Input: part model. Units: mm. Frame: model coordinates. Coordinates: 2 decimals unless noted, no trailing zeros. Order: outer loops, then holes, each group sorted by start corner. A loop starts at its lowest first (then second) coordinate and runs counter-clockwise, first axis right, second up. Notation, with made-up numbers: (-6.5, 14) -> (42.5, 14) arc R23 cw to (42.5, 30) -> close; hole circle Ø11 at (-6.5, -29). An arc over 180 degrees is marked (long way). Write each question's results on one line, items separated by ' | '.
```python
from build123d import *

# Parameters (mm, degrees)
F0_R     = 2.5527
F1_DEPTH = 6


with BuildPart() as f1:
    # F0 (on Right) → F1 (new body)
    with BuildSketch(Plane.YZ):
        with BuildLine():
            Line((-63.5, 177.8), (-114.3, 177.8))
            Line((-114.3, 177.8), (-114.3, 0))
            Line((-114.3, 0), (114.3, 0))
            Line((114.3, 0), (114.3, 177.8))
            Line((114.3, 177.8), (63.5, 177.8))
            ThreePointArc((63.5, 177.8), (0, 151.497439), (-63.5, 177.8))
        make_face()
        with Locations((-101.6, 12.7)):
            Circle(F0_R, mode=Mode.SUBTRACT)
        with Locations((-88.9, 12.7)):
            Circle(F0_R, mode=Mode.SUBTRACT)
        with Locations((-76.2, 12.7)):
            Circle(F0_R, mode=Mode.SUBTRACT)
        with Locations((-63.5, 12.7)):
            Circle(F0_R, mode=Mode.SUBTRACT)
        with Locations((-101.6, 25.4)):
            Circle(F0_R, mode=Mode.SUBTRACT)
        with Locations((-101.6, 38.1)):
            Circle(F0_R, mode=Mode.SUBTRACT)
        with Locations((-50.8, 12.7)):
            Circle(F0_R, mode=Mode.SUBTRACT)
        with Locations((-38.1, 12.7)):
            Circle(F0_R, mode=Mode.SUBTRACT)
        with Locations((-25.4, 12.7)):
            Circle(F0_R, mode=Mode.SUBTRACT)
        with Locations((-12.7, 12.7)):
            Circle(F0_R, mode=Mode.SUBTRACT)
        with Locations((-101.6, 50.8)):
            Circle(F0_R, mode=Mode.SUBTRACT)
        with Locations((-101.6, 63.5)):
            Circle(F0_R, mode=Mode.SUBTRACT)
        with Locations((-101.6, 76.2)):
            Circle(F0_R, mode=Mode.SUBTRACT)
        with Locations((0, 12.7)):
            Circle(F0_R, mode=Mode.SUBTRACT)
        with Locations((12.7, 12.7)):
            Circle(F0_R, mode=Mode.SUBTRACT)
        with Locations((25.4, 12.7)):
            Circle(F0_R, mode=Mode.SUBTRACT)
        with Locations((38.1, 12.7)):
            Circle(F0_R, mode=Mode.SUBTRACT)
        with Locations((50.8, 12.7)):
            Circle(F0_R, mode=Mode.SUBTRACT)
        with Locations((63.5, 12.7)):
            Circle(F0_R, mode=Mode.SUBTRACT)
        with Locations((76.2, 12.7)):
            Circle(F0_R, mode=Mode.SUBTRACT)
        with Locations((88.9, 12.7)):
            Circle(F0_R, mode=Mode.SUBTRACT)
        with Locations((101.6, 12.7)):
            Circle(F0_R, mode=Mode.SUBTRACT)
        with Locations((101.6, 25.4)):
            Circle(F0_R, mode=Mode.SUBTRACT)
        with Locations((101.6, 38.1)):
            Circle(F0_R, mode=Mode.SUBTRACT)
        with Locations((101.6, 50.8)):
            Circle(F0_R, mode=Mode.SUBTRACT)
        with Locations((101.6, 63.5)):
            Circle(F0_R, mode=Mode.SUBTRACT)
        with Locations((101.6, 76.2)):
            Circle(F0_R, mode=Mode.SUBTRACT)
        with Locations((-101.6, 88.9)):
            Circle(F0_R, mode=Mode.SUBTRACT)
        with Locations((-101.6, 101.6)):
            Circle(F0_R, mode=Mode.SUBTRACT)
        with Locations((-101.6, 114.3)):
            Circle(F0_R, mode=Mode.SUBTRACT)
        with Locations((-101.6, 127)):
            Circle(F0_R, mode=Mode.SUBTRACT)
        with Locations((-101.6, 139.7)):
            Circle(F0_R, mode=Mode.SUBTRACT)
        with Locations((-101.6, 152.4)):
            Circle(F0_R, mode=Mode.SUBTRACT)
        with Locations((-101.6, 165.1)):
            Circle(F0_R, mode=Mode.SUBTRACT)
        with Locations((101.6, 88.9)):
            Circle(F0_R, mode=Mode.SUBTRACT)
        with Locations((101.6, 101.6)):
            Circle(F0_R, mode=Mode.SUBTRACT)
        with Locations((101.6, 114.3)):
            Circle(F0_R, mode=Mode.SUBTRACT)
        with Locations((101.6, 127)):
            Circle(F0_R, mode=Mode.SUBTRACT)
        with Locations((101.6, 139.7)):
            Circle(F0_R, mode=Mode.SUBTRACT)
        with Locations((101.6, 152.4)):
            Circle(F0_R, mode=Mode.SUBTRACT)
        with Locations((101.6, 165.1)):
            Circle(F0_R, mode=Mode.SUBTRACT)
    extrude(amount=F1_DEPTH)


solid = f1.part
```
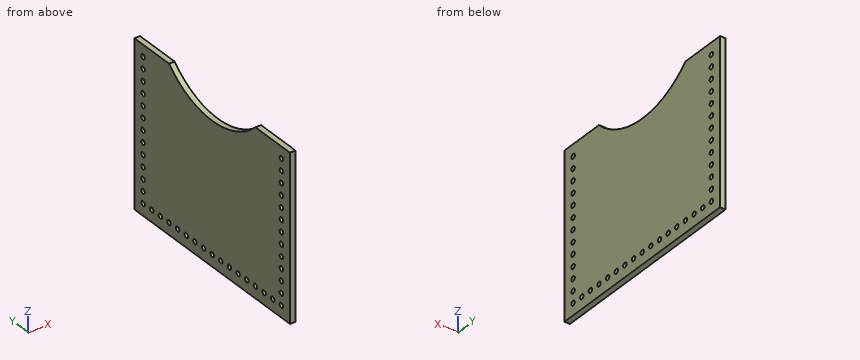
(1) Cut plane C-C, the plane y = -50.8. Return loops of the section in (x, z), plus the area to 3 significant figures.
Return value:
outline: (0, 0) -> (6, 0) -> (6, 10.15) -> (0, 10.15) -> close; (0, 15.25) -> (6, 15.25) -> (6, 167.25) -> (0, 167.25) -> close | area: 973 mm2
(2) Cut plane A-A, the plane z = 76.2. Return loops of the section in (x, y).
Return value:
outline: (0, -114.3) -> (6, -114.3) -> (6, -104.15) -> (0, -104.15) -> close; (0, -99.05) -> (6, -99.05) -> (6, 99.05) -> (0, 99.05) -> close; (0, 104.15) -> (6, 104.15) -> (6, 114.3) -> (0, 114.3) -> close
(3) Cut plane D-D, the plane x = 2.9. Count the separate pieces of the cut face and the enclosed holes in it, plus the area to 3 significant figures.
Return value:
separate pieces: 1 | enclosed holes: 41 | area: 37,500 mm2
(4) Pin query (flat end, axial travel): P1, Ø4, axis at y = -101.6, z = 127, coming from the +X side. Return the tip coordinate at first contact, or that it passes through.
Return value:
P1: through
(5) Line query: line 1 along Y through (x, z) = (4.35, 76); line 2 along Z through (x, y) = (2.65, -63.5); line 3 along Z through (x, y) = (1, 77.5). Output: solid intervals per line, ascending. Write a range as from..to.
Return value:
line 1: -114.3..-104.14, -99.06..99.06, 104.14..114.3 | line 2: 0..10.15, 15.25..177.8 | line 3: 0..10.5, 14.9..177.8
(6) Cut plane B-B, the plane y = 76.2. Return loops of the section in (x, z), plus the area to 3 significant figures.
Return value:
outline: (0, 0) -> (6, 0) -> (6, 10.15) -> (0, 10.15) -> close; (0, 15.25) -> (6, 15.25) -> (6, 177.8) -> (0, 177.8) -> close | area: 1,040 mm2
